Could you check a few things on this drawing? It's one solid part, dimensions in mm from its lowest x, y, z. A direction names the side the tool comes from. Give positions to 0.01 mm unless a question says otherwise; leave off trailing zeros. Loops run counter-clockwise (first coordinate to the right, second up) from the corner with the lowest first, then second, coordinate; pieces in that order, holes last. Notation, with made-up numbers: (-24, 27) -> (29, 27) arc R4 cw to (29, 32) -> close; hole circle Ø6 at (-28, 73). An arc over 180 degrees is marked (long way). Use CSV: the item, a comma, the result in double quotes.
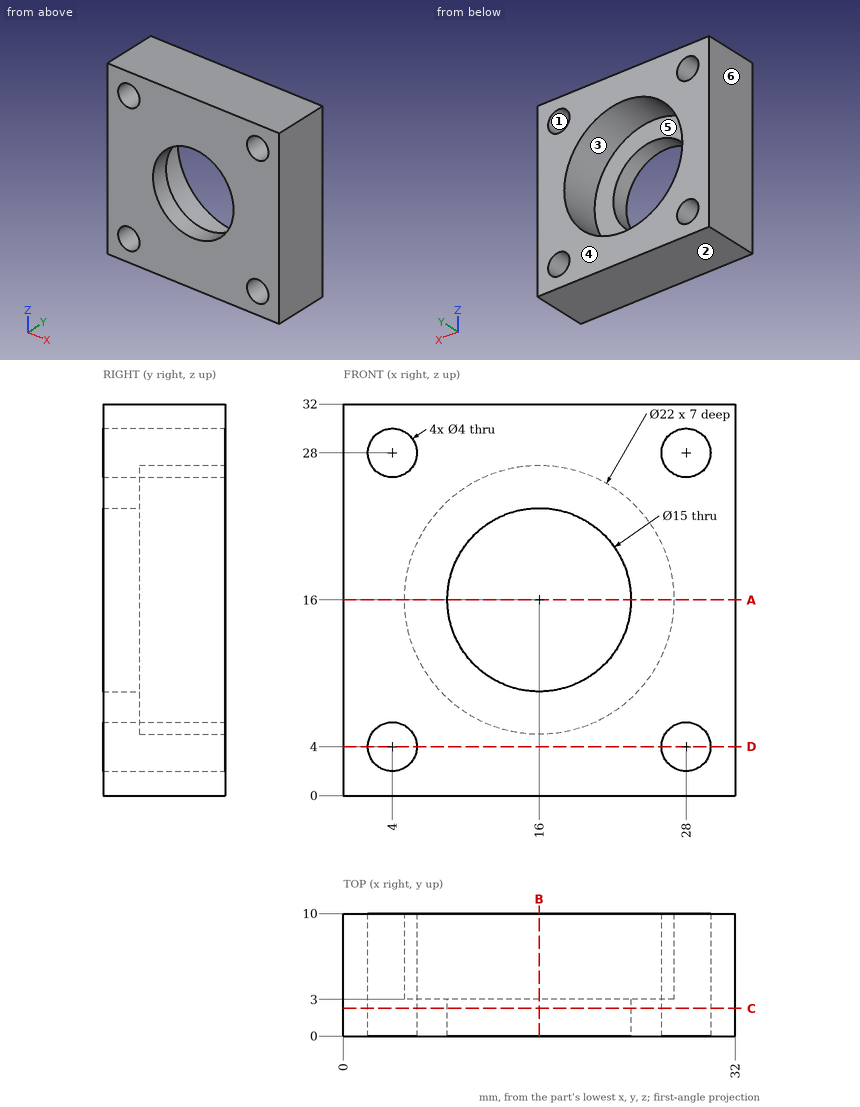
(1) If I drill on L1, parallel to X at y = 3.25, z = 28; L2, parallel to Z at x = 16, y = 8.25, over which ranges is the centre line in solid material (lowest first)? Write a range as from..to.
Answer sheet:
L1,"x = 0..2, 6..26, 30..32"
L2,"z = 0..5, 27..32"
(2) If we section it at A-A, the plane z = 16: Write out the boundary of the cut face in (x, y).
Answer sheet:
outline,"(0, 0) -> (8.5, 0) -> (8.5, 3) -> (5, 3) -> (5, 10) -> (0, 10) -> close; (23.5, 0) -> (32, 0) -> (32, 10) -> (27, 10) -> (27, 3) -> (23.5, 3) -> close"
(3) If we section it at B-B, the plane x = 16: Write out the boundary of the cut face in (y, z), then the cut area to 3 significant figures.
Answer sheet:
outline,"(0, 0) -> (10, 0) -> (10, 5) -> (3, 5) -> (3, 8.5) -> (0, 8.5) -> close; (0, 23.5) -> (3, 23.5) -> (3, 27) -> (10, 27) -> (10, 32) -> (0, 32) -> close"
area,"121 mm2"
(4) If we section it at C-C, the plane y = 2.25: Write out the boundary of the cut face in (x, z), then the cut area to 3 significant figures.
Answer sheet:
outline,"(0, 0) -> (32, 0) -> (32, 32) -> (0, 32) -> close; hole circle Ø4 at (4, 4); hole circle Ø4 at (4, 28); hole circle Ø15 at (16, 16); hole circle Ø4 at (28, 4); hole circle Ø4 at (28, 28)"
area,"797 mm2"
(5) Will this pin go through, and if not, where does the flat tip stop? pin 1 Ø17 at (x, z) = (16, 16) entering from +Y.
Answer sheet:
pin 1,"stops at y = 3"
(6) We'd pull the mould along Z, two halves only. Please class the marked faces 1, 2, 3 and 4: released by +Z, released by -Z, zero draft, split by the parting line, or undercut.
Answer sheet:
face 1,"undercut"
face 2,"released by -Z"
face 3,"undercut"
face 4,"zero draft"
(7) If we section it at D-D, the plane z = 4: Write out the boundary of the cut face in (x, y).
Answer sheet:
outline,"(0, 0) -> (2, 0) -> (2, 10) -> (0, 10) -> close; (6, 0) -> (26, 0) -> (26, 10) -> (6, 10) -> close; (30, 0) -> (32, 0) -> (32, 10) -> (30, 10) -> close"
(8) Which directions (+Z, -Z, +X, -X, +Y, -Y) give clear straight access to the entire face, cutting with the end or side of a thin tool? Please do the marked faces 5 and 6.
Answer sheet:
face 5,"+Y"
face 6,"+Z, -Z, -X, +Y, -Y"
